from build123d import *

# Parameters (mm, degrees)
ESQUISSE1_W             = 46
ESQUISSE1_H             = 47
ESQUISSE1_R             = 2.2
BOSS_EXTRU_1_DEPTH      = 5
BOSS_EXTRU_2_START      = -5
BOSS_EXTRU_2_DEPTH      = 45.3
ESQUISSE3_R             = 6.5
ESQUISSE3_R_2           = 1.6
ENL_V_MAT_EXTRU_1_DEPTH = 15
ESQUISSE4_W             = 57
ESQUISSE4_H             = 5
BOSS_EXTRU_3_DEPTH      = 20
ESQUISSE7_W             = 57
ESQUISSE7_H             = 5
BOSS_EXTRU_4_DEPTH      = 16
ESQUISSE8_R             = 18.55
ENL_V_MAT_EXTRU_3_DEPTH = 52
ENL_V_MAT_EXTRU_4_DEPTH = 10
ENL_V_MAT_EXTRU_5_DEPTH = 10
BOSS_EXTRU_6_DEPTH      = 5.5
BOSS_EXTRU_7_START      = -5.5
BOSS_EXTRU_7_DEPTH      = 5.5
ESQUISSE14_R            = 2.2
ENL_V_MAT_EXTRU_6_DEPTH = 10


with BuildPart() as part:
    # Esquisse1 → Boss.-Extru.1 (new body)
    with BuildSketch(Plane(origin=(0, 0, 0), x_dir=(1, 0, 0), z_dir=(0, 1, 0))):
        Rectangle(ESQUISSE1_W, ESQUISSE1_H)
        with Locations(Location((-15, 13.5, 0), (0, 0, 270))):
            Circle(ESQUISSE1_R, mode=Mode.SUBTRACT)
        with Locations(Location((-15, -16.5, 0), (0, 0, 270))):
            Circle(ESQUISSE1_R, mode=Mode.SUBTRACT)
        with Locations(Location((15, -16.5, 0), (0, 0, 270))):
            Circle(ESQUISSE1_R, mode=Mode.SUBTRACT)
        with Locations(Location((15, 13.5, 0), (0, 0, 270))):
            Circle(ESQUISSE1_R, mode=Mode.SUBTRACT)
    extrude(amount=BOSS_EXTRU_1_DEPTH)

    # Esquisse2 → Boss.-Extru.2 (add)
    with BuildSketch(Plane.XZ.offset(BOSS_EXTRU_2_START)):
        Polygon((-28.5, -27.5), (-28.5, 23.5), (-23, 23.5), (-23, -23.5), (23, -23.5), (23, 23.5), (28.5, 23.5), (28.5, -27.5), align=None)
    extrude(amount=BOSS_EXTRU_2_DEPTH)

    # Esquisse3 → Enlèv. mat.-Extru.1 (cut)
    with BuildSketch(Plane.XY.offset(-23.5)):
        with Locations((0, -10)):
            Circle(ESQUISSE3_R)
        with Locations((7.75, -30.423393759)):
            Circle(ESQUISSE3_R_2)
        with Locations((-7.75, -30.423393759)):
            Circle(ESQUISSE3_R_2)
        with Locations((-15.5, -17)):
            Circle(ESQUISSE3_R_2)
        with Locations((-7.75, -3.576606241)):
            Circle(ESQUISSE3_R_2)
        with Locations((7.75, -3.576606241)):
            Circle(ESQUISSE3_R_2)
        with Locations((15.5, -17)):
            Circle(ESQUISSE3_R_2)
    extrude(amount=-ENL_V_MAT_EXTRU_1_DEPTH, mode=Mode.SUBTRACT)

    # Esquisse4 → Boss.-Extru.3 (add)
    with BuildSketch(Plane(origin=(0, 0, -27.5), x_dir=(-1, 0, 0), z_dir=(0, 0, -1))):
        with Locations((0, -42.8)):
            Rectangle(ESQUISSE4_W, ESQUISSE4_H)
    extrude(amount=-BOSS_EXTRU_3_DEPTH)

    # Esquisse7 → Boss.-Extru.4 (add)
    with BuildSketch(Plane(origin=(0, 5, 0), x_dir=(1, 0, 0), z_dir=(0, 1, 0))):
        with Locations((0, -26)):
            Rectangle(ESQUISSE7_W, ESQUISSE7_H)
    extrude(amount=-BOSS_EXTRU_4_DEPTH)

    # Esquisse8 → Enlèv. mat.-Extru.3 (cut)
    with BuildSketch(Plane.XY.offset(28.5)):
        with Locations((0, -17)):
            Circle(ESQUISSE8_R)
    extrude(amount=-ENL_V_MAT_EXTRU_3_DEPTH, mode=Mode.SUBTRACT)

    # Esquisse10 → Enlèv. mat.-Extru.4 (cut)
    with BuildSketch(Plane(origin=(28.5, 0, 0), x_dir=(0, 0, -1), z_dir=(1, 0, 0))):
        Polygon((-23.5, -11), (7.5, -40.3), (-23.5, -40.3), align=None)
    extrude(amount=-ENL_V_MAT_EXTRU_4_DEPTH, mode=Mode.SUBTRACT)

    # Esquisse11 → Enlèv. mat.-Extru.5 (cut)
    with BuildSketch(Plane.ZY.offset(28.5)):
        Polygon((23.5, -11), (-7.5, -40.3), (23.5, -40.3), align=None)
    extrude(amount=-ENL_V_MAT_EXTRU_5_DEPTH, mode=Mode.SUBTRACT)

    # Esquisse12 → Boss.-Extru.6 (add)
    with BuildSketch(Plane.ZY.offset(28.5)):
        Polygon((-7.5, -45.3), (28.5, -11), (23.5, -11), (-7.5, -40.3), align=None)
    extrude(amount=-BOSS_EXTRU_6_DEPTH)

    # Esquisse13 → Boss.-Extru.7 (add)
    with BuildSketch(Plane(origin=(28.5, 0, 0), x_dir=(0, 0, -1), z_dir=(1, 0, 0)).offset(BOSS_EXTRU_7_START)):
        Polygon((-28.5, -11), (7.5, -45.3), (7.5, -40.3), (-23.5, -11), align=None)
    extrude(amount=BOSS_EXTRU_7_DEPTH)

    # Esquisse14 → Enlèv. mat.-Extru.6 (cut)
    with BuildSketch(Plane.XZ.offset(45.3)):
        with Locations(Location((-14.5, -17.5, 0), (0, 0, 270))):
            Circle(ESQUISSE14_R)
        with Locations(Location((14.5, -17.5, 0), (0, 0, 270))):
            Circle(ESQUISSE14_R)
    extrude(amount=-ENL_V_MAT_EXTRU_6_DEPTH, mode=Mode.SUBTRACT)


solid = part.part
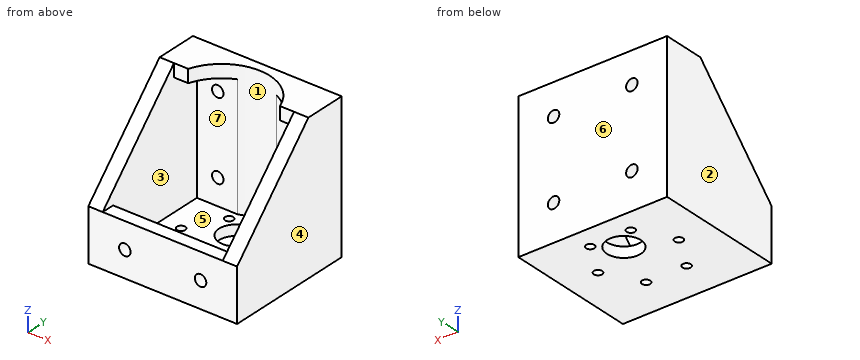
Here's how the part is built. I have some questions about the finished solid (model axes, mm). Face numbers are marked on the shaded views. A direction names the side the tool comes from. Round coordinates to 2 decimals unless told otherwise and drop trailing zeros. Write each loop counter-clockwise with the first axis right and the second up, starting at its lowest first coordinate (ties: lowest second). Pieces come first, ordered by that corner, then holes.
1. If we mould it in two halves opening along Y, with no side actions, what happens to the marked faces 4, 5, 6 and 7? For each: released by +Y, released by -Y, zero draft, split by the parting line, or undercut.
2. Suppose I cut it at D-D (x = -20). List the corners of the cut face in (y, z) for me.
3. Suppose I cut it at B-B (x = 0). List the corners of the cut face in (y, z) for me, and give its area (3 significant figures).
4. For the marked faces 1, 2 and 3, which set-ups out of +Z, -Z, +X, -X, +Y, -Y let a thin tool reach every point of the face, with its end or its side?
5. Suppose I cut it at C-C (z = 17.5). List the corners of the cut face in (x, y) for me, and give its area (3 significant figures).
6. I need wall thicknesses on L1, parallel to X at y = 3.3, z = 16.5; L2, parallel to Y at x = -7.75, z = -25.7; L3, parallel to X at y = -15.5, z = -6. Which ranges of each line are inside material? Lowest first, please.
7. Will these pins go through, and if not, where does the flat tip stop? pin 1 Ø21 at (x, y) = (-0.5, -29) entering from +Z; pin 2 Ø1.5 at (x, z) = (-20.5, 26.5) entering from -Y; pin 3 Ø2 at (x, z) = (15.5, 6.5) entering from -Y.
8. Suppose I cut it at A-A (z = -13.5). List the corners of the cut face in (x, y) for me.
Answer sheet:
1. face 4: zero draft
1. face 5: undercut
1. face 6: released by +Y
1. face 7: undercut
2. outline: (-45.3, -27.5) - (5, -27.5) - (5, 28.5) - (-11, 28.5) - (-11, 23.5) - (0, 23.5) - (0, -23.5) - (-40.3, -23.5) - (-40.3, -7.5) - (-45.3, -7.5) - close
3. outline: (-45.3, -27.5) - (-16.5, -27.5) - (-16.5, -23.5) - (-40.3, -23.5) - (-40.3, -7.5) - (-45.3, -7.5) - close; (-3.5, -27.5) - (5, -27.5) - (5, 28.5) - (1.55, 28.5) - (1.55, -23.5) - (-3.5, -23.5) - close
3. area: 409 mm2
4. face 1: +Z
4. face 2: +Z, -Z, -X, +Y, -Y
4. face 3: none
5. outline: (-28.5, -21.48) - (-23, -21.48) - (-23, 0) - (-16.96, 0) - (-16.96, 5) - (-28.5, 5) - close; (-13.04, 0) - (-7.42, 0) arc R18.55 cw to (7.42, 0) - (13.04, 0) - (13.04, 5) - (-13.04, 5) - close; (16.96, 0) - (23, 0) - (23, -21.48) - (28.5, -21.48) - (28.5, 5) - (16.96, 5) - close
5. area: 467 mm2
6. L1: x = -28.5 to -17.2, -12.8 to 12.8, 17.2 to 28.5
6. L2: y = -45.3 to -32.02, -28.82 to -5.18, -1.98 to 5
6. L3: x = -28.5 to -23, 23 to 28.5
7. pin 1: stops at z = -23.5
7. pin 2: stops at y = -11
7. pin 3: stops at y = 0
8. outline: (-28.5, -45.3) - (28.5, -45.3) - (28.5, 5) - (17.2, 5) - (17.2, 0) - (23, 0) - (23, -40.3) - (-23, -40.3) - (-23, 0) - (-17.2, 0) - (-17.2, 5) - (-28.5, 5) - close; (-12.8, 0) - (-7.42, 0) arc R18.55 cw to (7.42, 0) - (12.8, 0) - (12.8, 5) - (-12.8, 5) - close
